from build123d import *

# Parameters (mm, degrees)
F0_R      = 1.65
F0_R_2    = 2
F1_DEPTH  = 3.7
F2_R      = 4.15
F2_R_2    = 2
F2_R_3    = 1.65
F3_DEPTH  = 7.5
F4_R      = 2
F5_R      = 1
F6_R      = 2.9
F7_DEPTH  = 3.3
F8_R      = 1
F10_DEPTH = 11.0010001
F11_SIZE  = 3


with BuildPart() as f1:
    # F0 (on Front) → F1 (new body)
    with BuildSketch(Plane.XZ):
        with BuildLine():
            Line((5, 23), (-1, 23))
            Line((-1, 23), (-1, 10.4))
            add(Edge.make_bspline(
                [(-1, 10.4), (-1.2111639775, 7.9330686148), (-2.6557673414, 5.8471197981), (-4.3304576575, 4.3515548571)],
                knots=[0, 0, 0, 0, 6.6865737794, 6.6865737794, 6.6865737794, 6.6865737794], degree=3))
            ThreePointArc((-4.3304576575, 4.3515548571), (-5.5635670417, 2.6652064856), (-6, 0.6222048076))
            Line((-6, 0.6222048076), (-6, -23))
            Line((-6, -23), (6, -23))
            Line((6, -23), (6, 1.2846305262))
            ThreePointArc((6, 1.2846305262), (5.9790845004, 1.6382624525), (5.9166296405, 1.9869634531))
            add(Edge.make_bspline(
                [(5, 10.4), (5.3525537919, 5.8237470378), (5.0164384354, 5.7252537292), (5.9166296405, 1.9869634531)],
                knots=[0, 0, 0, 0, 8.5585174857, 8.5585174857, 8.5585174857, 8.5585174857], degree=3))
            Line((5, 10.4), (5, 23))
        make_face()
        with Locations((1, -17.45)):
            Circle(F0_R, mode=Mode.SUBTRACT)
        with Locations((0, -1.77)):
            Circle(F0_R_2, mode=Mode.SUBTRACT)
    extrude(amount=F1_DEPTH)

    # F2 (on face) → F3 (join)
    with BuildSketch(Plane.XZ.offset(3.7)):
        with Locations((0, -1.77)):
            Circle(F2_R)
        with Locations((0, -1.77)):
            Circle(F2_R_2, mode=Mode.SUBTRACT)
        with BuildLine():
            Line((-6, -12.9), (-6, -23))
            Line((-6, -23), (6, -23))
            Line((6, -23), (6, -12.9))
            ThreePointArc((6, -12.9), (0, -14.3674374053), (-6, -12.9))
        make_face()
        with Locations((1, -17.45)):
            Circle(F2_R_3, mode=Mode.SUBTRACT)
        Polygon((5, 23), (-1, 23), (-1, 11.03), (5, 10.4), (5, 10.44), align=None)
    extrude(amount=F3_DEPTH)

    # F4
    f4_edges = [f1.edges().sort_by_distance(p)[0] for p in [
        (5, -5.6, 23),
        (-1, -5.6, 23),
    ]]
    fillet(f4_edges, radius=F4_R)

    # F5
    f5_edges = [f1.edges().sort_by_distance(p)[0] for p in [
        (-1, -7.45, 11.03),
        (5, -7.45, 10.4),
        (6, -7.45, -12.9),
        (-6, -7.45, -12.9),
    ]]
    fillet(f5_edges, radius=F5_R)

    # F6 (on face) → F7 (cut)
    with BuildSketch(Plane.XZ.offset(11.2)):
        with Locations((1, -17.45)):
            Circle(F6_R)
    extrude(amount=-F7_DEPTH, mode=Mode.SUBTRACT)

    # F8
    f8_edges = [f1.edges().sort_by_distance(p)[0] for p in [
        (-4.15, -11.2, -1.77),
    ]]
    fillet(f8_edges, radius=F8_R)

    # F9 (on face) → F10 (cut, through all)
    with BuildSketch(Plane.YZ.offset(5)):
        with BuildLine():
            Line((-5.3, 14.0104973894), (-5.3, 17.0104973894))
            ThreePointArc((-5.3, 17.0104973894), (-7.3, 19.0104973894), (-9.3, 17.0104973894))
            Line((-9.3, 17.0104973894), (-9.3, 14.0104973894))
            ThreePointArc((-9.3, 14.0104973894), (-7.3, 12.0104973894), (-5.3, 14.0104973894))
        make_face()
    extrude(amount=-F10_DEPTH, mode=Mode.SUBTRACT)

    # F11
    f11_edges = [f1.edges().sort_by_distance(p)[0] for p in [
        (-6, -5.6, -23),
    ]]
    chamfer(f11_edges, length=F11_SIZE)


solid = f1.part
Geometry check sheet. Reference: the model listing, model coordinates, mm. A direction names the side the tool comes from. Coordinates: 2 decimals unless noted, no trailing zeros. Order: outer loops, then holes, each group sorted by start corner. A loop starts at its lowest first (then second) coordinate and runs counter-clockwise, first axis right, second up. Notation, with made-up numbers: M 11.25,-12 L 31.25,-12 A23 cw 31.25,-2 Z; hole C 63,25.25 d1. An arc over 180 degrees is marked long. Use CSV: the item, a comma, the result in double quotes.
Item 1: Mould release check, pull along Z, two halves, no side actions. Record for faces 1 (the flat face through (-0.1, -11.2, -20.3)), 2 (the flat face through (4, -3.7, -4)), 3 (the flat face through (-4, -6, -22)), 4 (the cylindrical face through (5.58, -7.5, -13.63)): pulls with the +Z half, pulls with the -Z half, needs draft (parallel to the pull), parting line crosses it, or undercut.
Returned:
face 1,"needs draft"
face 2,"undercut"
face 3,"pulls with the -Z half"
face 4,"undercut"
Item 2: Tool access check on faces 5 (the cylindrical face through (-5.58, -7.5, -13.63)), 6 (the flat face through (2, -7.9, -19)), 7 (the cylindrical face through (2.04, -7.34, 12.01)). Record the directions out of +Z, -Z, +X, -X, +Y, -Y that give a thin tool (end or side, any length) a straight path to the whole face; none if there is none.
Returned:
face 5,"+Z, -Y"
face 6,"-Y"
face 7,"+X, -X"
Item 3: Thickness scan on line 1 along Y through (x, z) = (1, 14.5); line 2 along Z through (x, y) = (-1.5, -8.5); line 3 along X through (y, z) = (-3.25, -17.45). Record the ranges inside material, lowest first.
Returned:
line 1,"y = -11.2 to -9.3, -5.3 to 0"
line 2,"z = -23 to -18.92, -15.98 to -14.28, -5.64 to -3.09, -0.45 to 2.1"
line 3,"x = -6 to -0.65, 2.65 to 6"
Item 4: Cross-section at A-A on z = -17.45. Record the cut outline in (x, y).
Returned:
outline,"M -6,-11.2 L -1.9,-11.2 L -1.9,-7.9 L -0.65,-7.9 L -0.65,0 L -6,0 Z; M 2.65,-7.9 L 3.9,-7.9 L 3.9,-11.2 L 6,-11.2 L 6,0 L 2.65,0 Z"
Item 5: Gauge pin test, flat ends, axial feed: pin 1 Ø5 at (y, z) = (-2.5, 7.5) entering from -X; pin 2 Ø1.7 at (x, z) = (0, -16.5) entering from -Y; pin 3 Ø3.5 at (x, z) = (0, -1.77) entering from +Y; pin 4 Ø5 at (x, z) = (1, -17.45) entering from +Y. Record the tip position at first contact, or that the pin passes through.
Returned:
pin 1,"stops at x = -3.66"
pin 2,"stops at y = -7.9"
pin 3,"passes through"
pin 4,"stops at y = 0"
Item 6: Cross-section at D-D on y = -2.75. Give the number of separate pieces and of enclosed holes in the cut face, then the cut area to 3 significant figures.
Returned:
separate pieces,"1"
enclosed holes,"2"
area,"418 mm2"
Item 7: Cross-section at C-C on z = -1.77. Record the cut outline in (x, y), then the cut area to 3 significant figures.
Returned:
outline,"M -6,-3.7 L -4.15,-3.7 L -4.15,-10.2 A1 ccw -3.15,-11.2 L -2,-11.2 L -2,0 L -6,0 Z; M 2,-11.2 L 3.15,-11.2 A1 ccw 4.15,-10.2 L 4.15,-3.7 L 6,-3.7 L 6,0 L 2,0 Z"
area,"61.4 mm2"
Item 8: Cross-section at B-B on y = -7.3. Record the cut outline in (x, z).
Returned:
outline,"M -6,-20 L -3,-23 L 6,-23 L 6,-14.44 A1 ccw 4.64,-13.51 A13 cw -4.64,-13.51 A1 ccw -6,-14.44 Z; C 0,-1.77 d8.3; M -1,11.93 A1 ccw -0.1,10.94 L 3.9,10.52 A1 ccw 5,11.51 L 5,12.01 L -1,12.01 Z; M -1,19.01 L 5,19.01 L 5,21 A2 ccw 3,23 L 1,23 A2 ccw -1,21 Z; hole C 0,-1.77 d4; hole C 1,-17.45 d3.3"
